Geometry: see drawing. Coordinates: mm, zero at the bounding-box minimum. A direction names the side the tool comes from. Coordinates: 2 decimals unless noted, no trailing zeros. Order: outer loops, then holes, each group sorted by start corner. A loop starts at its lowest first (then second) coordinate and runs counter-clockwise, first axis right, second up. Notation, with made-up numbers: M 3.5,75 L 17.5,75 A17 cw 17.5,107 Z; hole C 15.5,-6 d11. An arc over 180 degrees is marked long. One line per item, written item: value.
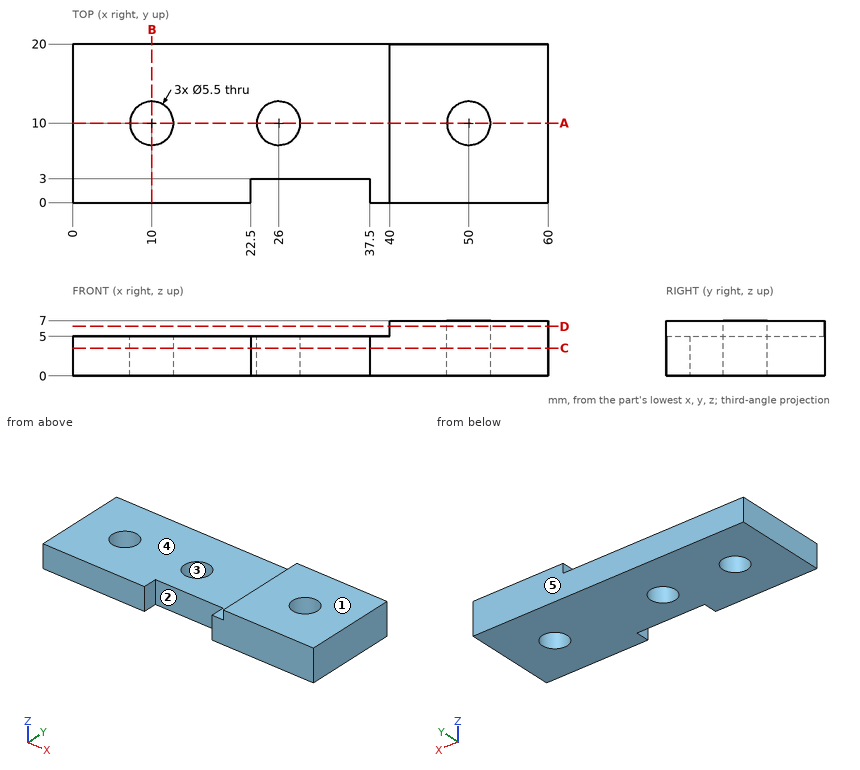
(1) Cut plane A-A on y = 10. Output: boundary loops of the cut face in (x, z).
Data:
outline: M 0,0 L 7.25,0 L 7.25,5 L 0,5 Z; M 12.75,0 L 23.25,0 L 23.25,5 L 12.75,5 Z; M 28.75,0 L 47.25,0 L 47.25,7 L 40,7 L 40,5 L 28.75,5 Z; M 52.75,0 L 60,0 L 60,7 L 52.75,7 Z
(2) Access query for the marked faces 1 and 2. Directions: +Z, -Z, +X, -X, +Y, -Y. A direction counts if a zero-diameter tool reaches every point of the face in a straight line with its end or side. Return the directions, or none.
Data:
face 1: +Z, +X, -X, +Y, -Y
face 2: +Z, -Z, -Y
(3) Cut plane B-B on x = 10. Output: boundary loops of the cut face in (y, z), plus the area to 3 significant figures.
Data:
outline: M 0,0 L 7.25,0 L 7.25,5 L 0,5 Z; M 12.75,0 L 20,0 L 20,5 L 12.75,5 Z
area: 72.5 mm2
(4) Draft query along Y for the marked faces 3, 4 and 5. Return one class per face: released by +Y, released by -Y, zero draft, split by the parting line, or undercut.
Data:
face 3: undercut
face 4: zero draft
face 5: released by +Y
(5) First-contact query: pin 1 (3.5 mm diameter, centred on x = 26, y = 10, fed in from +Z); pin 2 (10 mm diameter, centred on x = 11.5, y = 8, fed in from +Z); pin 3 (4 mm diameter, centred on x = 21.5, y = 10.5, fed in from -Z); pin 4 (2.5 mm diameter, centred on x = 29, z = 2, fed in from -Y). Flat tips, straight axial feed; report the tip coordinate or a pass-through.
Data:
pin 1: passes through
pin 2: stops at z = 5
pin 3: stops at z = 0
pin 4: stops at y = 3
(6) Cut plane C-C on z = 3.5. Output: boundary loops of the cut face in (x, y), plus the area to 3 significant figures.
Data:
outline: M 0,0 L 22.5,0 L 22.5,3 L 37.5,3 L 37.5,0 L 60,0 L 60,20 L 0,20 Z; hole C 10,10 d5.5; hole C 26,10 d5.5; hole C 50,10 d5.5
area: 1,080 mm2
(7) Cut plane D-D on z = 6.25. Output: boundary loops of the cut face in (x, y), plus the area to 3 significant figures.
Data:
outline: M 40,0 L 60,0 L 60,20 L 40,20 Z; hole C 50,10 d5.5
area: 376 mm2
(8) Ray query, line 1 (X direction, y = 10, z = 3.35); line 2 (Y direction, x = 50, z = 2.5); line 3 (X direction, y = 11, z = 1.75). Return the intervals inside material, ascending. Write a range as from..to.
Data:
line 1: x = 0..7.25, 12.75..23.25, 28.75..47.25, 52.75..60
line 2: y = 0..7.25, 12.75..20
line 3: x = 0..7.44, 12.56..23.44, 28.56..47.44, 52.56..60
